Geometry: final body of the model. Coordinates: model frame, mm. Coordinates: 2 decimals unless noted, no trailing zeros. Order: outer loops, then holes, each group sorted by start corner. A loop starts at its lowest first (then second) coordinate and runs counter-clockwise, first axis right, second up. Notation, with made-up numbers: M 77,-31 L 127,-31 A16 cw 127,-2 Z; hole C 0.5,35 d9. An arc over 180 degrees is marked long. One line per question, with ' | ' between items.
from build123d import *

# Parameters (mm, degrees)
F1_DEPTH = 60
F3_DEPTH = 75
F4_R     = 15
F5_DEPTH = 25


# Not quite as in the source:
# - a feature names something its author has since deleted; it is built from what else it names


with BuildPart() as f1:
    # F0 (on Front) → F1 (new body, symmetric)
    with BuildSketch(Plane.XZ):
        with BuildLine():
            ThreePointArc((-50, 196.9523800313), (0, 203.2), (50, 196.9523800313))
            Line((50, 196.9523800313), (35, 220.857542129))
            ThreePointArc((35, 220.857542129), (33.1846822218, 222.5753691641), (30.7647349749, 223.2))
            Line((30.7647349749, 223.2), (-30.7647349749, 223.2))
            ThreePointArc((-30.7647349749, 223.2), (-33.1846822218, 222.5753691641), (-35, 220.857542129))
            Line((-35, 220.857542129), (-50, 196.9523800313))
        make_face()
    extrude(amount=F1_DEPTH, both=True)

    # F2 (on Right) → F3 (cut, symmetric)
    with BuildSketch(Plane.YZ):
        with BuildLine():
            Line((60, 223.2), (46.5543481195, 223.2))
            ThreePointArc((46.5543481195, 223.2), (49.3915485081, 222.3170734697), (51.2267330988, 219.980117582))
            Line((51.2267330988, 219.980117582), (60, 196.9523800313))
            Line((60, 196.9523800313), (60, 223.2))
        make_face()
        with BuildLine():
            ThreePointArc((-51.2267330988, 219.980117582), (-49.3915485081, 222.3170734697), (-46.5543481195, 223.2))
            Line((-46.5543481195, 223.2), (-60, 223.2))
            Line((-60, 223.2), (-60, 196.9523800313))
            Line((-60, 196.9523800313), (-51.2267330988, 219.980117582))
        make_face()
    extrude(amount=F3_DEPTH, both=True, mode=Mode.SUBTRACT)

    # F4 (on face) → F5 (cut)
    with BuildSketch(Plane.XY.offset(223.2)):
        with Locations((0, 15)):
            Circle(F4_R)
    extrude(amount=-F5_DEPTH, mode=Mode.SUBTRACT)


solid = f1.part
1. Material intervals for line 1 (Y direction, x = -6.5, z = 217.5); line 2 (Y direction, x = 0, z = 218.5); line 3 (X direction, y = 15, z = 210.25), sorted ascending. Write a range as [from, to].
Response values:
line 1: y = [-52.17, 1.48], [28.52, 52.17] | line 2: y = [-51.79, 0], [30, 51.79] | line 3: x = [-41.66, -15], [15, 41.66]
2. Section B-B, the plane z = 200.5. Output: boundary loops of the cut face in (x, y) (3 decimals).
Response values:
outline: M -47.774,-58.648 L -33.015,-58.648 L -33.015,58.648 L -47.774,58.648 Z; M 33.015,-58.648 L 47.774,-58.648 L 47.774,58.648 L 33.015,58.648 Z
3. Section A-A, the plane y = 15. Output: boundary loops of the cut face in (x, z), and give its area (3 significant figures).
Response values:
outline: M -50,196.95 A203.2 cw -15,202.65 L -15,223.2 L -30.76,223.2 A5 ccw -35,220.86 Z; M 15,202.65 A203.2 cw 50,196.95 L 35,220.86 A5 ccw 30.76,223.2 L 15,223.2 Z | area: 1,170 mm^2
4. Section C-C, the plane y = -21.5. Output: boundary loops of the cut face in (x, z).
Response values:
outline: M -50,196.95 A203.2 cw 50,196.95 L 35,220.86 A5 ccw 30.76,223.2 L -30.76,223.2 A5 ccw -35,220.86 Z
5. Draft query along X for faces 1 (the face through (-33.154, -0.711, 222.592)), 2 (the face through (-0.7, 55.55, 208.63)), 3 (the face through (-3.252, 0.357, 213.067)), 4 (the face through (-0.7, -0.8, 203.2)). Return one class per face: pulls with the +X half, pulls with the -X half, needs draft (parallel to the pull), parting line crosses it, or undercut.
Response values:
face 1: pulls with the -X half | face 2: needs draft | face 3: undercut | face 4: undercut
6. Section D-D, the plane x = 0. Output: boundary loops of the cut face in (y, z), and give its area (3 significant figures).
Response values:
outline: M -57.62,203.2 L 0,203.2 L 0,223.2 L -46.55,223.2 A5 ccw -51.23,219.98 Z; M 30,203.2 L 57.62,203.2 L 51.23,219.98 A5 ccw 46.55,223.2 L 30,223.2 Z | area: 1,550 mm^2
7. Pin query (flat end, axial travel): P1, Ø4, axis at x = -20.5, z = 219.5, coming from the -Y side; P2, Ø12, axis at x = -1.5, y = 9, coming from the -Z side; P3, Ø4, axis at x = 10.5, z = 204, coming from the -Y side; P4, Ø12, axis at y = 9.5, z = 220.5, coming from the +X side. Return the tip coordinate at first contact, or that it passes through.
Response values:
P1: stops at y = -52.17 | P2: passes through | P3: stops at y = -57.76 | P4: stops at x = 38.99
